Input: part model. Units: mm. Frame: model coordinates. Face numbers are marked on the shaded views. A direction names the side the tool comes from. Round coordinates to 2 decimals unless told otherwise and drop trailing zeros. Write each loop counter-clockwise with the first axis right and the second up, starting at its lowest first coordinate (ties: lowest second). Pieces come first, ordered by that corner, then holes. Notation, with made-up numbers: (-38.75, -10) -> (0.25, -10) arc R31 ccw to (0.25, 22) -> close; hole circle Ø10 at (64.25, 60.25). An arc over 180 degrees is marked (long way). Write item = value, one per line.
```python
from build123d import *

# Parameters (mm, degrees)
F1_DEPTH = 58.42


with BuildPart() as f1:
    # F0 (on Front) → F1 (new body)
    with BuildSketch(Plane.XZ):
        Polygon((-353.620197, 171.341745), (-366.987277, 145.822746), (-363.949285, 129.417699), (-362.734098, 77.16454), (-365.164497, 58.936687), (-356.658164, 39.493647), (-303.189818, 39.493647), (-298.329045, 46.784793), (-291.037924, 47.99998), (-225.417685, 78.379726), (-215.696165, 66.227833), (-174.379712, 66.227833), (-168.303753, 57.7215), (-165.873379, 41.924046), (-184.101232, 18.835421), (-203.544272, -10.329113), (-198.683499, -40.708859), (-180.455646, -58.936712), (-167.088566, -58.936712), (-158.582233, -45.569632), (-157.367046, -32.202526), (-139.139219, -1.822806), (-131.848073, 0.607593), (-131.848073, 4.253154), (-114.835407, 24.91138), (-68.658207, 24.91138), (-56.506313, 33.417713), (-0.607593, 33.417713), (-87.493653, -164.050624), (-75.341759, -178.632891), (60.759492, -178.632891), (140.962024, -1.215187), (162.835438, -1.215187), (174.987331, 20.658226), (190.784785, 32.81012), (210.227824, 37.670867), (226.025304, 38.886054), (226.025304, 32.81012), (317.164517, 32.81012), (329.31641, 54.683533), (326.886037, 76.556946), (351.189823, 76.556946), (359.696156, 81.417693), (366.987303, 92.3544), (366.987303, 109.367066), (359.696156, 117.873399), (351.189823, 121.518959), (328.101223, 121.518959), (339.03793, 130.025292), (339.03793, 134.88604), (334.177183, 143.392373), (334.177183, 162.835412), (323.240476, 162.835412), (309.873371, 176.202492), (-131.240479, 178.632866), (-131.240479, 171.341745), align=None)
    extrude(amount=F1_DEPTH)


solid = f1.part
```
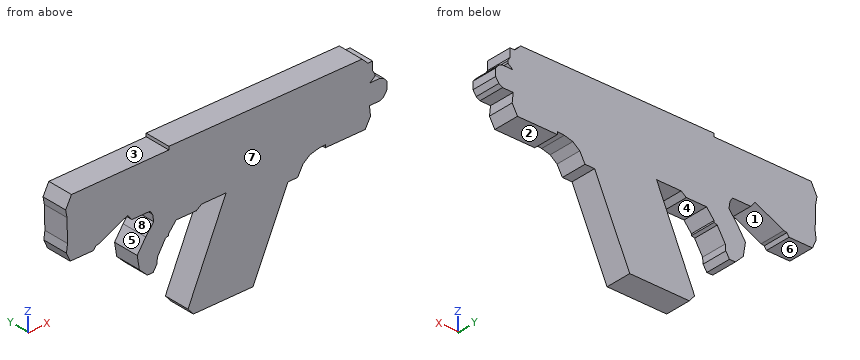
1) Access query for the marked faces 1, 2, 3, 4 and 5. Directions: +Z, -Z, +X, -X, +Y, -Y. A direction counts if a zero-diameter tool reaches every point of the face in a straight line with its end or side. Return the directions, or none.
Solutions:
face_1 = -Z, +Y, -Y
face_2 = -Z, +X, +Y, -Y
face_3 = +Z, -X, +Y, -Y
face_4 = +Y, -Y
face_5 = -X, +Y, -Y
2) Line query: L1, parallel to Z at x = -317, y = -50; L2, parallel to Z at x = -213.5, y = -51; L3, parallel to X at y = -25, z = 29.5. Output: solid intervals per line, ascending. Write a range as from..to.
Solutions:
L1 = 39.49..171.34
L2 = 66.23..171.34
L3 = -175.68..-62.1, -2.33..186.48
3) Draft query along Z for the marked faces 6, 7 and 8. Return one class per face: +Z half, -Z half, draft (parallel to the pull), parting line (faces both ways), or undercut.
Solutions:
face_6 = -Z half
face_7 = draft
face_8 = undercut
4) First-contact query: P1, Ø8, axis at x = 102, y = -33, coming from the -Z side; P2, Ø1.5, axis at y = -32.5, z = 93.5, coming from the -X side; P3, Ø4, axis at y = -17.5, z = -65.5, coming from the +X side. Flat tips, straight axial feed; report the tip coordinate or a pass-through.
Solutions:
P1 = -96.25
P2 = -363.13
P3 = 112.81
5) Cut plane B-B (x = 152.5). Return the cut outline in (y, z), and give its area (3 significant figures).
Solutions:
outline = (-58.42, -1.22) -> (0, -1.22) -> (0, 177.07) -> (-58.42, 177.07) -> close
area = 10,400 mm^2
6) Cut plane A-A (z = -72). Return the cut outline in (x, y).
Solutions:
outline = (-46.99, -58.42) -> (108.96, -58.42) -> (108.96, 0) -> (-46.99, 0) -> close
